from build123d import *

# Parameters (mm, degrees)
SKETCH1_W           = 150
SKETCH1_H           = 150
BOSS_EXTRUDE1_DEPTH = 0.5
SKETCH2_W           = 150
SKETCH2_H           = 150
SKETCH2_W_2         = 146
SKETCH2_H_2         = 146
BOSS_EXTRUDE2_DEPTH = 15
SKETCH6_W           = 150
SKETCH6_H           = 150
SKETCH6_W_2         = 146
SKETCH6_H_2         = 146
BOSS_EXTRUDE4_DEPTH = 135
SKETCH7_W           = 150
SKETCH7_H           = 150
BOSS_EXTRUDE5_DEPTH = 1.5
SKETCH8_R           = 5
CUT_EXTRUDE1_DEPTH  = 226.333641519
SKETCH9_R           = 5
CUT_EXTRUDE2_DEPTH  = 226.333641519


with BuildPart() as part:
    # Sketch1 → Boss-Extrude1 (new body)
    with BuildSketch(Plane(origin=(0, 0, 0), x_dir=(1, 0, 0), z_dir=(0, 1, 0))):
        Rectangle(SKETCH1_W, SKETCH1_H)
    extrude(amount=BOSS_EXTRUDE1_DEPTH)

    # Sketch2 → Boss-Extrude2 (add)
    with BuildSketch(Plane(origin=(0, 0.5, 0), x_dir=(1, 0, 0), z_dir=(0, 1, 0))):
        Rectangle(SKETCH2_W, SKETCH2_H)
        Rectangle(SKETCH2_W_2, SKETCH2_H_2, mode=Mode.SUBTRACT)
    extrude(amount=BOSS_EXTRUDE2_DEPTH)

    # Sketch6 → Boss-Extrude4 (add)
    with BuildSketch(Plane(origin=(0, 15.5, 0), x_dir=(1, 0, 0), z_dir=(0, 1, 0))):
        Rectangle(SKETCH6_W, SKETCH6_H)
        Rectangle(SKETCH6_W_2, SKETCH6_H_2, mode=Mode.SUBTRACT)
    extrude(amount=BOSS_EXTRUDE4_DEPTH)

    # Sketch7 → Boss-Extrude5 (add)
    with BuildSketch(Plane.XZ):
        Rectangle(SKETCH7_W, SKETCH7_H)
    extrude(amount=BOSS_EXTRUDE5_DEPTH)

    # Sketch8 → Cut-Extrude1 (cut, through all)
    with BuildSketch(Plane(origin=(0, 0, -75), x_dir=(-1, 0, 0), z_dir=(0, 0, -1))):
        with Locations((0, 74.5)):
            Circle(SKETCH8_R)
    extrude(amount=-CUT_EXTRUDE1_DEPTH, mode=Mode.SUBTRACT)

    # Sketch9 → Cut-Extrude2 (cut, through all)
    with BuildSketch(Plane.ZY.offset(75)):
        with Locations((0, 64.5)):
            Circle(SKETCH9_R)
    extrude(amount=-CUT_EXTRUDE2_DEPTH, mode=Mode.SUBTRACT)


solid = part.part
Could you check a few things on this model? Use its own coordinates, in mm. A direction names the side the tool comes from. Give positions to 0.01 mm unless a question says otherwise; leave off trailing zeros. Order: outer loops, then holes, each group sorted by start corner. A loop starts at its lowest first (then second) coordinate and runs counter-clockwise, first axis right, second up. Notation, with made-up numbers: M -8,-14 L 8,-14 A30 ccw 8,16 Z; hole C 11.25,-34.75 d6. An arc over 180 degrees is marked long. One line per question, with ' | ' between items.
1. I want a section at A-A (x = 0). List the corners of the cut face in (y, z) for me, and give its area (3 significant figures).
Results:
outline: M -1.5,-75 L 69.5,-75 L 69.5,-73 L 0.5,-73 L 0.5,73 L 69.5,73 L 69.5,75 L -1.5,75 Z; M 79.5,-75 L 150.5,-75 L 150.5,-73 L 79.5,-73 Z; M 79.5,73 L 150.5,73 L 150.5,75 L 79.5,75 Z | area: 860 mm²
2. If I drill on line 1 (Z direction, x = 14, y = 124.5); line 2 (Y direction, x = -74, z = 0), over which ranges is the centre line in solid material (lowest first)?
Results:
line 1: -75 to -73, 73 to 75 | line 2: -1.5 to 59.5, 69.5 to 150.5
3. I want a section at C-C (z = 0). List the corners of the cut face in (x, y) for me, and give its area (3 significant figures).
Results:
outline: M -75,-1.5 L 75,-1.5 L 75,59.5 L 73,59.5 L 73,0.5 L -73,0.5 L -73,59.5 L -75,59.5 Z; M -75,69.5 L -73,69.5 L -73,150.5 L -75,150.5 Z; M 73,69.5 L 75,69.5 L 75,150.5 L 73,150.5 Z | area: 860 mm²
4. We'd pull the mould along X, two halves only. Please class faces 3 (the face through (75, 76, -1)), 4 (the face through (-73, 74, 1)), 5 (the face through (16, 76, -75)), 6 (the face through (1.08, 69.62, -74.01)): +X half, -X half, draft (parallel to the pull), parting line (faces both ways), or undercut.
Results:
face 3: +X half | face 4: undercut | face 5: draft | face 6: undercut
5. I'm going to push flat-ended pins straight in: pin 1 (10 mm diameter, centred on x = -14.5, z = 32.5, fed in from +Y); pin 2 (6 mm diameter, centred on x = 0, y = 74.5, fed in from +Z). Where does each tip first touch, or does it pass through?
Results:
pin 1: y = 0.5 | pin 2: through
6. For faces 1 (the face through (73, 74, 1)), 2 (the face through (-75, 76, -1)), which set-ups out of +Z, -Z, +X, -X, +Y, -Y let a thin tool reach every point of the face, with its end or its side?
Results:
face 1: +Y | face 2: +Z, -Z, -X, +Y, -Y
7. I want a section at D-D (x = 38.5). List the corners of the cut face in (y, z) for me.
Results:
outline: M -1.5,-75 L 150.5,-75 L 150.5,-73 L 0.5,-73 L 0.5,73 L 150.5,73 L 150.5,75 L -1.5,75 Z
8. I want a section at B-B (y = 64.5). List the corners of the cut face in (x, z) for me.
Results:
outline: M -75,-75 L 75,-75 L 75,-5 L 73,-5 L 73,-73 L -73,-73 L -73,-5 L -75,-5 Z; M -75,5 L -73,5 L -73,73 L 73,73 L 73,5 L 75,5 L 75,75 L -75,75 Z
